from build123d import *

# Parameters (mm, degrees)
F0_W     = 306
F0_H     = 127
F0_R     = 1.6
F0_W_2   = 89
F0_H_2   = 8
F0_W_3   = 11
F0_H_3   = 35
F0_W_4   = 54
F0_H_4   = 14
F0_W_5   = 32
F0_W_6   = 16.6
F0_H_5   = 17.1
F0_W_7   = 5
F0_H_6   = 18
F0_W_8   = 41
F0_H_7   = 9
F1_DEPTH = 1
F2_W     = 148.235004
F2_H     = 139.296211
F3_DEPTH = 12.5


with BuildPart() as f1:
    # F0 (on Top) → F1 (new body)
    with BuildSketch(Plane.XY):
        Rectangle(F0_W, F0_H)
        with Locations((-150, -52.5)):
            Circle(F0_R, mode=Mode.SUBTRACT)
        with Locations((0, -58.5)):
            Circle(F0_R, mode=Mode.SUBTRACT)
        with Locations((150, -52.5)):
            Circle(F0_R, mode=Mode.SUBTRACT)
        with Locations((85.5, -8.5)):
            Rectangle(F0_W_2, F0_H_2, mode=Mode.SUBTRACT)
        with Locations((-150, 0)):
            Circle(F0_R, mode=Mode.SUBTRACT)
        with Locations((-140, 25.5)):
            Rectangle(F0_W_3, F0_H_3, mode=Mode.SUBTRACT)
        with Locations((-150, 52.5)):
            Circle(F0_R, mode=Mode.SUBTRACT)
        with Locations((-119, 55)):
            Rectangle(F0_W_4, F0_H_4, mode=Mode.SUBTRACT)
        with Locations((-75, 55)):
            Rectangle(F0_W_5, F0_H_4, mode=Mode.SUBTRACT)
        with Locations((-19.5, 52.65)):
            Rectangle(F0_W_6, F0_H_5, mode=Mode.SUBTRACT)
        Circle(F0_R, mode=Mode.SUBTRACT)
        with Locations((150, 0)):
            Circle(F0_R, mode=Mode.SUBTRACT)
        with Locations((114.5, 20.5)):
            Rectangle(F0_W_7, F0_H_6, mode=Mode.SUBTRACT)
        with Locations((0, 58.5)):
            Circle(F0_R, mode=Mode.SUBTRACT)
        with Locations((32.5, 57.5)):
            Rectangle(F0_W_8, F0_H_7, mode=Mode.SUBTRACT)
        with Locations((77.5, 57.5)):
            Rectangle(F0_W_8, F0_H_7, mode=Mode.SUBTRACT)
        with Locations((150, 52.5)):
            Circle(F0_R, mode=Mode.SUBTRACT)
        with Locations((122.5, 57.5)):
            Rectangle(F0_W_8, F0_H_7, mode=Mode.SUBTRACT)
    extrude(amount=F1_DEPTH)

    # F2 (on Top) → F3 (cut, symmetric)
    with BuildSketch(Plane.XY):
        with Locations((-81.938947, 0.248301)):
            Rectangle(F2_W, F2_H)
    extrude(amount=F3_DEPTH, both=True, mode=Mode.SUBTRACT)


solid = f1.part
CAD build for the part. Positions are in the model's coordinates, mm. Round coordinates to 2 decimals unless told otherwise and drop trailing zeros. Write each loop counter-clockwise with the first axis right and the second up, starting at its lowest first coordinate (ties: lowest second). Pieces come first, ordered by that corner, then holes.
(1) Slice it at A-A, the plane x = 71.5. Write the cut outline in (y, z), and give its area (3 significant figures).
(2) Slice it at B-B, the plane z = 0.85. Count the separate pieces of the cut face and the enclosed holes in it, and give its area (3 significant figures).
(3) Mould opens along Y. For faces 1 (the face through (-1.27, -0.97, 0.49)), 2 (the face through (71, 1, 1)), 3 (the face through (151.48, 51.89, 0.49)) say: pulls with the +Y half, pulls with the -Y half, needs draft (parallel to the pull), parting line crosses it, or undercut.
(4) Probe line 1 along X through (y, z) = (55.5, 0.35); line 2 along Y through (x, z) = (116, 0.4); line 3 along Y through (x, z) = (106, 0.2). List the from-to ranges inside material, lowest first.
From the geometry:
1. outline: (-63.5, 0) - (-12.5, 0) - (-12.5, 1) - (-63.5, 1) - close; (-4.5, 0) - (53, 0) - (53, 1) - (-4.5, 1) - close; (62, 0) - (63.5, 0) - (63.5, 1) - (62, 1) - close
1. area: 110 mm2
2. separate pieces: 1
2. enclosed holes: 11
2. area: 18,500 mm2
3. face 1: undercut
3. face 2: needs draft
3. face 3: undercut
4. line 1: x = -7.82 to 12, 53 to 57, 98 to 102, 143 to 153
4. line 2: y = -63.5 to -12.5, -4.5 to 11.5, 29.5 to 53, 62 to 63.5
4. line 3: y = -63.5 to -12.5, -4.5 to 53, 62 to 63.5
